Here's how the part is built. I have some questions about the finished solid (model axes, mm). A direction names the side the tool comes from. Give positions to 0.01 mm unless a question says otherwise; leave off trailing zeros. Loops run counter-clockwise (first coordinate to the right, second up) from the corner with the lowest first, then second, coordinate; pieces in that order, holes last. Notation, with made-up numbers: (11, -34) - (25, -34) arc R24 ccw to (25, -20) - close; hole circle Ø1 at (77.25, 52.25). An arc over 180 degrees is marked (long way). Use a Markdown table: item, result.
from build123d import *

# Parameters (mm, degrees)
SKETCH3_W               = 120
SKETCH3_H               = 80
BOSS_EXTRUDE1_DEPTH     = 20
CUT_EXTRUDE3_DEPTH      = 129.062484749
CUT_EXTRUDE3_DEPTH_BACK = 120
SKETCH5_W               = 6
SKETCH5_H               = 6
BOSS_EXTRUDE2_DEPTH     = 120
SKETCH6_W               = 120
SKETCH6_H               = 3.448417199
CUT_EXTRUDE4_DEPTH      = 10


with BuildPart() as part:
    # Sketch3 → Boss-Extrude1 (new body)
    with BuildSketch(Plane(origin=(0, 0, 0), x_dir=(1, 0, 0), z_dir=(0, 1, 0))):
        Rectangle(SKETCH3_W, SKETCH3_H)
    extrude(amount=BOSS_EXTRUDE1_DEPTH)

    # Sketch4 → Cut-Extrude3 (cut, two sides: drawn at the far end of the back side and taken through both)
    with BuildSketch(Plane(origin=(60, 0, 0), x_dir=(0, 0, -1), z_dir=(1, 0, 0)).offset(-CUT_EXTRUDE3_DEPTH_BACK)):
        Polygon((-40, 20), (-40, 0), (-39.971354494, 0), (40, 20), align=None)
    extrude(amount=CUT_EXTRUDE3_DEPTH + CUT_EXTRUDE3_DEPTH_BACK, mode=Mode.SUBTRACT)

    # Sketch5 → Boss-Extrude2 (add)
    with BuildSketch(Plane(origin=(60, 0, 0), x_dir=(0, 0, -1), z_dir=(1, 0, 0))):
        with Locations((7.014322753, -3)):
            Rectangle(SKETCH5_W, SKETCH5_H)
    extrude(amount=-BOSS_EXTRUDE2_DEPTH)

    # Sketch6 → Cut-Extrude4 (cut)
    with BuildSketch(Plane(origin=(0, 9.407996907, 2.352841706), x_dir=(1, 0, 0), z_dir=(0, 0.9701220558238487, 0.2426173876788501))):
        with Locations((0, -37.052883997)):
            Rectangle(SKETCH6_W, SKETCH6_H)
    extrude(amount=-CUT_EXTRUDE4_DEPTH, mode=Mode.SUBTRACT)


solid = part.part
(1) On a 3-axis mill with a long thin cutter (end or side, diameter ignored), from which of +Z, -Z, +X, -X, +Y, -Y can I reach the whole of each face in a straight line? I mean faces 1 (the face through (1, -3, -10.014)), 2 (the face through (-1, 0, 16)), 3 (the face through (1, -6, -7)). Say none if no direction works.
A:
| item | result |
|---|---|
| face 1 | -Z, +X, -X, -Y |
| face 2 | +Z, +X, -X, -Y |
| face 3 | +Z, -Z, +X, -X, -Y |
(2) Suppose I cut it at B-B on y = 6.25. Write out the boundary of the cut face in (x, z), plus the area to 3 significant figures.
A:
| item | result |
|---|---|
| outline | (-60, -40) - (60, -40) - (60, 14.98) - (-60, 14.98) - close |
| area | 6,600 mm2 |
(3) Will these pins go through, and if not, where does the flat tip stop? pin 1 (5 mm diameter, centred on x = 44.5, z = 1.5, fed in from -Y); pin 2 (3 mm diameter, centred on x = -28.5, y = -2.5, fed in from +Z); pin 3 (5 mm diameter, centred on x = 25, y = -3.5, fed in from -Z).
A:
| item | result |
|---|---|
| pin 1 | y = 0 |
| pin 2 | z = -4.01 |
| pin 3 | z = -10.01 |
(4) Suppose I cut it at C-C on z = 21.5. Write out the boundary of the cut face in (x, y).
A:
| item | result |
|---|---|
| outline | (-60, 0) - (60, 0) - (60, 4.62) - (-60, 4.62) - close |
(5) Suppose I cut it at A-A on x = 3. Write out the boundary of the cut face in (y, z), plus the area to 3 significant figures.
A:
| item | result |
|---|---|
| outline | (-6, -10.01) - (0, -10.01) - (0, -40) - (20, -40) - (0.84, 36.63) - (0, 36.42) - (0, -4.01) - (-6, -4.01) - close |
| area | 834 mm2 |
(6) If I drill on line 1 (Z direction, x = -36, y = -0.75); line 2 (Z direction, x = -2.5, y = 0.75); line 3 (Y direction, x = 13.5, z = 31.5), over which ranges is the centre line in solid material (lowest first)?
A:
| item | result |
|---|---|
| line 1 | -10.01 to -4.01 |
| line 2 | -40 to 36.6 |
| line 3 | 0 to 2.12 |
